from build123d import *

# Parameters (mm, degrees)
ESQUISSE1_R             = 70
BOSS_EXTRU_2_DEPTH      = 100
ESQUISSE2_R             = 50
ENL_V_MAT_EXTRU_2_DEPTH = 95
ESQUISSE4_R             = 50
ENL_V_MAT_EXTRU_3_DEPTH = 101


with BuildPart() as part:
    # Esquisse1 → Boss.-Extru.2 (new body)
    with BuildSketch(Plane(origin=(0, 0, 0), x_dir=(1, 0, 0), z_dir=(0, 1, 0))):
        with BuildLine():
            Line((1070.306926615, 30.095541494), (63.200145428, 30.095541494))
            ThreePointArc((63.200145428, 30.095541494), (68.278877334, 15.427083652), (70, 0))
            ThreePointArc((70, 0), (68.278877334, -15.427083652), (63.200145428, -30.095541494))
            Line((63.200145428, -30.095541494), (1070.306926615, -30.095541494))
            ThreePointArc((1070.306926615, -30.095541494), (1063.507072043, 0), (1070.306926615, 30.095541494))
        make_face()
        Circle(ESQUISSE1_R)
        with Locations((1133.507072043, 0)):
            Circle(ESQUISSE1_R)
    extrude(amount=BOSS_EXTRU_2_DEPTH)

    # Esquisse2 → Enlèv. mat.-Extru.2 (cut)
    with BuildSketch(Plane(origin=(0, 100, 0), x_dir=(1, 0, 0), z_dir=(0, 1, 0))):
        Circle(ESQUISSE2_R)
    extrude(amount=-ENL_V_MAT_EXTRU_2_DEPTH, mode=Mode.SUBTRACT)

    # Esquisse4 → Enlèv. mat.-Extru.3 (cut, through all)
    with BuildSketch(Plane(origin=(0, 100, 0), x_dir=(1, 0, 0), z_dir=(0, 1, 0))):
        with Locations((1133.507072043, 0)):
            Circle(ESQUISSE4_R)
    extrude(amount=-ENL_V_MAT_EXTRU_3_DEPTH, mode=Mode.SUBTRACT)


solid = part.part
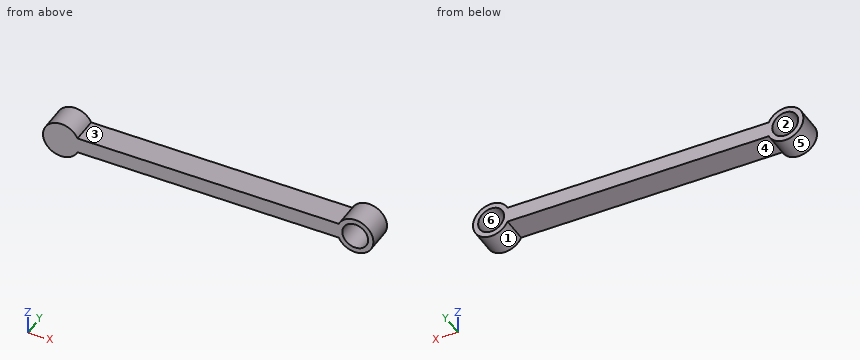
Design review of the part built by this model. Coordinates are the model's own, in mm. Face numbers are marked on the shaded views. A direction names the side the tool comes from. Give positions to 0.01 mm unless a question says otherwise; leave off trailing zeros. Order: outer loops, then holes, each group sorted by start corner. A loop starts at its lowest first (then second) coordinate and runs counter-clockwise, first axis right, second up.
1. Add section A-A, the plane z = 0. State the section outline as (x, y) points.
Solution:
outline: (-70, 0) - (1083.51, 0) - (1083.51, 100) - (50, 100) - (50, 5) - (-50, 5) - (-50, 100) - (-70, 100) - close; (1183.51, 0) - (1203.51, 0) - (1203.51, 100) - (1183.51, 100) - close
2. Tool access review of the marked faces 1, 2 and 3: name each direction out of +Z, -Z, +X, -X, +Y, -Y from which nothing blocks a thin tool from reaching the whole face with its end or side.
Solution:
face 1: +Y, -Y
face 2: +Y
face 3: +Z, +Y, -Y
3. Add section C-C, the plane y = 76. State the section outline as (x, z) points, then the cut area to 3 significant figures.
Solution:
outline: (63.2, -30.1) - (1070.31, -30.1) arc R70 ccw (long way) to (1070.31, 30.1) - (63.2, 30.1) arc R70 ccw (long way) to start; hole circle Ø100 at (0, 0); hole circle Ø100 at (1133.51, 0)
area: 75,100 mm2
4. Add section B-B, the plane x = 0. State the section outline as (y, z) points, then the cut area to 3 significant figures.
Solution:
outline: (0, -70) - (100, -70) - (100, -50) - (5, -50) - (5, 50) - (100, 50) - (100, 70) - (0, 70) - close
area: 4,500 mm2
5. To check wall thickness, follow L1, parallel to Z at x = 0, y = 81; L2, parallel to X at y = 51, z = -35; L3, parallel to Z at x = 280, y = 15. State the ranges of each line that lie inside material, in increasing order.
Solution:
L1: z = -70 to -50, 50 to 70
L2: x = -60.62 to -35.71, 35.71 to 60.62, 1072.89 to 1097.8, 1169.21 to 1194.13
L3: z = -30.1 to 30.1
6. Add section D-D, the plane x = 664.5. State the section outline as (y, z) points.
Solution:
outline: (0, -30.1) - (100, -30.1) - (100, 30.1) - (0, 30.1) - close
7. Mouldability with a two-part tool opening along Z and no side actions: class the marked faces 4, 5 and 6 as +Z half, -Z half, draft (parallel to the pull), parting line (faces both ways), or undercut.
Solution:
face 4: -Z half
face 5: parting line
face 6: undercut
8. For pin 1 Ø5 at (y, z) = (46.5, -55.5) entering from +X; pin 2 Ø1.5 at (y, z) = (63.5, 30.5) entering from -X; pin 3 Ø12 at (x, z) = (427, -37.5) entering from +Y; pin 4 Ø4 at (y, z) = (42.5, -22.5) entering from -X, all flat-tipped, find the tip position at first contact; note any pin that passes through.
Solution:
pin 1: stops at x = 1179.23
pin 2: stops at x = -63.36
pin 3: passes through
pin 4: stops at x = -66.93
